The listing builds one solid part. Answer for the finished solid, in the listing's coordinates (mm). Give positions to 0.01 mm unless a question says otherwise; leave off trailing zeros. Write each loop counter-clockwise with the first axis right and the second up, starting at its lowest first coordinate (ties: lowest second). Pieces come first, ordered by that corner, then holes. Notation, with made-up numbers: (14, -40) - (66, -40) arc R27 ccw to (66, -1) - close; hole circle Ø7 at (10.25, -37). An arc over 180 degrees is marked (long way). Answer in a Markdown table with one row per item. Add a question column.
from build123d import *

# Parameters (mm, degrees)
SKETCH1_W            = 304.8
SKETCH1_H            = 304.8
BOSS_EXTRUDE1_DEPTH  = 2.9972
SKETCH2_W            = 38.1
SKETCH2_H            = 38.1
CUT_EXTRUDE1_DEPTH   = 2.9972
LPATTERN1_COUNT      = 3
LPATTERN1_PITCH      = 88.9
LPATTERN1_COUNT_DIR2 = 2
LPATTERN1_PITCH_DIR2 = 63.5


with BuildPart() as part:
    # Sketch1 → Boss-Extrude1 (new body)
    with BuildSketch(Plane(origin=(0, 0, 0), x_dir=(1, 0, 0), z_dir=(0, 1, 0))):
        Rectangle(SKETCH1_W, SKETCH1_H)
    extrude(amount=BOSS_EXTRUDE1_DEPTH)

    # Sketch2 → Cut-Extrude1 (cut)
    with BuildSketch(Plane(origin=(0, 2.9972, 0), x_dir=(1, 0, 0), z_dir=(0, 1, 0))):
        with Locations((-88.9, 88.9)):
            Rectangle(SKETCH2_W, SKETCH2_H)
    cut_extrude1 = extrude(amount=-CUT_EXTRUDE1_DEPTH, mode=Mode.SUBTRACT)

    # LPattern1: Cut-Extrude1 3 × 2
    with Locations(*[(i * LPATTERN1_PITCH, 0, j * LPATTERN1_PITCH_DIR2) for i in range(LPATTERN1_COUNT) for j in range(LPATTERN1_COUNT_DIR2) if (i, j) != (0, 0)]):
        add(cut_extrude1, mode=Mode.SUBTRACT)


solid = part.part
1. Section C-C (x = 5.5) is taken. Give the vertices of the cut face in (y, z), and give its area (3 significant figures).
2. Section A-A (z = -104) is taken. Give the vertices of the cut face in (x, y).
3. Straight lines are drawn through the part: L1, parallel to Z at x = 19, y = 1.8; L2, parallel to X at y = 1.1, z = -11. For each, find the intervals that lie inside material, in ascending order. Write a range as [from, to].
4. Section B-B (y = 2.5) is taken. Give the vertices of the cut face in (x, z).
Geometry check:
| question | item | result |
|---|---|---|
| 1 | outline | (0, -152.4) - (3, -152.4) - (3, -107.95) - (0, -107.95) - close; (0, -69.85) - (3, -69.85) - (3, -44.45) - (0, -44.45) - close; (0, -6.35) - (3, -6.35) - (3, 152.4) - (0, 152.4) - close |
| 1 | area | 685 mm² |
| 2 | outline | (-152.4, 0) - (-107.95, 0) - (-107.95, 3) - (-152.4, 3) - close; (-69.85, 0) - (-19.05, 0) - (-19.05, 3) - (-69.85, 3) - close; (19.05, 0) - (69.85, 0) - (69.85, 3) - (19.05, 3) - close; (107.95, 0) - (152.4, 0) - (152.4, 3) - (107.95, 3) - close |
| 3 | L1 | [-152.4, -107.95], [-69.85, -44.45], [-6.35, 152.4] |
| 3 | L2 | [-152.4, -107.95], [-69.85, -19.05], [19.05, 69.85], [107.95, 152.4] |
| 4 | outline | (-152.4, -152.4) - (152.4, -152.4) - (152.4, 152.4) - (-152.4, 152.4) - close; hole (-107.95, -107.95) - (-69.85, -107.95) - (-69.85, -69.85) - (-107.95, -69.85) - close; hole (-107.95, -44.45) - (-69.85, -44.45) - (-69.85, -6.35) - (-107.95, -6.35) - close; hole (-19.05, -107.95) - (19.05, -107.95) - (19.05, -69.85) - (-19.05, -69.85) - close; hole (-19.05, -44.45) - (19.05, -44.45) - (19.05, -6.35) - (-19.05, -6.35) - close; hole (69.85, -107.95) - (107.95, -107.95) - (107.95, -69.85) - (69.85, -69.85) - close; hole (69.85, -44.45) - (107.95, -44.45) - (107.95, -6.35) - (69.85, -6.35) - close |
